Autodesk Inventor part; units mm, degrees
ref_plane "Work Plane1" through (0, -22.925, 3.175) normal (1, 0, 0) x (0, 0, -1)
ref_plane "Work Plane2" through (-20.675, -22.925, -45) normal (0, 0, -1) x (1, 0, 0)
ref_plane "YZ Plane" through (0, 0, 0) normal (1, 0, 0) x (0, 1, 0)
sketch "Sketch1" plane through (0, 0, 0) normal (0, 0, 1) x (1, 0, 0)
  circle A0 centre (0, 0) radius 14.925 construction
  line L0 (-5.7359, -22.925) -> (4.2584, -22.925) construction
  line L1 (0, -14.925) -> (3.9694, -14.925) construction
  line L2 (-17.5, 17.075) -> (17.5, 17.075)
  line L3 (17.5, 17.075) -> (17.5, -22.925)
  line L4 (17.5, -22.925) -> (-17.5, -22.925)
  line L5 (-17.5, -22.925) -> (-17.5, 17.075)
  line L6 (0, 31.425) -> (0, -35.6875)
  line L7 (20.675, 21.8375) -> (20.675, -26.1)
  line L8 (20.675, -26.1) -> (-20.675, -26.1)
  line L9 (-20.675, -26.1) -> (-20.675, 21.8375)
  line L10 (-17.5, 17.075) -> (-19.0875, 17.075)
  line L11 (-19.0875, 17.075) -> (-19.0875, 20.25)
  line L12 (17.5, 17.075) -> (19.0875, 17.075)
  line L13 (19.0875, 17.075) -> (19.0875, 20.25)
  line L14 (17.5, 20.25) -> (17.5, 21.8375)
  line L15 (-17.5, 20.25) -> (-17.5, 21.8375)
  line L16 (-19.0875, 20.25) -> (-17.5, 20.25)
  line L17 (-17.5, 21.8375) -> (-20.675, 21.8375)
  line L18 (19.0875, 20.25) -> (17.5, 20.25)
  line L19 (17.5, 21.8375) -> (20.675, 21.8375)
  line L20 (-17.5, 21.8375) -> (17.5, 21.8375)
  dimension "d0" = 29.85
  dimension "d1" = 8
  dimension "d2" = 40
  dimension "d3" = 35
  dimension "d5" = 3.175
  dimension "d6" = 3.175
  dimension "d7" = 3.175
  dimension "d10" = 3.175
  dimension "d11" = 1.5875
  dimension "d12" = 1.5875
extrude "Extrusion1" add sketch "Sketch1" against normal blind 90 contours L5 L4 L6 L8 L9 L17 L15 L16 L11 L10 | L12 L13 L18 L14 L19 L7 L8 L6 L4 L3
extrude "Extrusion2" add sketch "Sketch1" along normal blind 3.175 contours L2 L6 L4 L5 | L5 L4 L6 L8 L9 L17 L15 L16 L11 L10 | L2 L3 L4 L6 | L12 L13 L18 L14 L19 L7 L8 L6 L4 L3
sketch "Sketch2" plane through (0, 0, -90) normal (0, 0, -1) x (-1, 0, 0)
  line L0 (19.0875, 17.075) -> (17.5, 17.075)
  line L1 (17.5, 17.075) -> (17.5, -22.925)
  line L2 (17.5, -22.925) -> (-17.5, -22.925)
  line L3 (-17.5, -22.925) -> (-17.5, 17.075)
  line L4 (-17.5, 17.075) -> (-19.0875, 17.075)
  line L5 (-19.0875, 17.075) -> (-19.0875, 20.25)
  line L6 (-19.0875, 20.25) -> (-17.5, 20.25)
  line L7 (-17.5, 20.25) -> (-17.5, 21.8375)
  line L8 (-17.5, 21.8375) -> (-20.675, 21.8375)
  line L9 (-20.675, 21.8375) -> (-20.675, -26.1)
  line L10 (-20.675, -26.1) -> (20.675, -26.1)
  line L11 (20.675, -26.1) -> (20.675, 21.8375)
  line L12 (20.675, 21.8375) -> (17.5, 21.8375)
  line L13 (17.5, 21.8375) -> (17.5, 20.25)
  line L14 (17.5, 20.25) -> (19.0875, 20.25)
  line L15 (19.0875, 20.25) -> (19.0875, 17.075)
  line L16 (-17.5, 21.8375) -> (17.5, 21.8375)
  line L17 (-17.5, 20.25) -> (17.5, 20.25)
  line L18 (-17.5, 17.075) -> (17.5, 17.075)
  point P0 (0, 0)
extrude "Extrusion3" add sketch "Sketch2" along normal blind 3.175
extrude "Extrusion4" cut sketch "Sketch2" along normal blind 1.5875 contours L0 L18 L4 L5 L6 L17 L14 L15
sketch "Sketch3" plane through (-17.5, -22.925, 0) normal (0, 1, 0) x (1, 0, 0)
  line L0 (-3.175, 93.175) -> (-3.175, -3.175)
  line L1 (38.175, 93.175) -> (-3.175, 93.175)
  line L2 (38.175, 93.175) -> (38.175, -3.175)
  line L3 (-3.175, -3.175) -> (38.175, -3.175)
  line L4 (-3.175, 93.175) -> (-3.175, -3.175) construction
  line L5 (-3.175, 45) -> (38.175, 45) construction
  line L6 (38.175, 93.175) -> (38.175, -3.175) construction
  line L7 (-3.175, -3.175) -> (38.175, -3.175) construction
  line L8 (17.5, -3.175) -> (17.5, 93.175) construction
  line L9 (38.175, 93.175) -> (-3.175, 93.175) construction
  circle A0 centre (17.5, 46.03) radius 9.75
  circle A1 centre (17.5, 46.03) radius 12.75 construction
  line L10 (17.5, 58.78) -> (17.5, 55.78) construction
  line L11 (17.5, 57.28) -> (18.611, 57.28) construction
  point P0 (17.5, 0)
  dimension "d22" = 19.5
  dimension "d23" = 25.5
  dimension "d21" = 1.03
extrude "Extrusion5" cut sketch "Sketch3" against normal up to next contours A0
hole "Hole1" at (0, -22.925, -57.28) direction (0, -1, 0) diameter 2 depth 8 tip angle 118
ref_plane "Work Plane1" through (0, -22.925, 3.175) normal (1, 0, 0) x (0, 0, -1)
ref_plane "Work Plane2" through (-20.675, -22.925, -45) normal (0, 0, -1) x (1, 0, 0)
pattern_circular "Circular Pattern1" count 8 over 360 about axis through (0, -26.1, -46.03) along (0, 1, 0) of "Hole1"
sketch "Sketch4" plane through (-17.5, 21.8375, -90) normal (0, 1, 0) x (1, 0, 0)
  circle A0 centre (25.455, -36.015) radius 1
  circle A1 centre (28.75, -43.97) radius 1
  circle A2 centre (25.455, -51.925) radius 1
  circle A3 centre (17.5, -55.22) radius 1
  circle A4 centre (9.545, -51.925) radius 1
  circle A5 centre (6.25, -43.97) radius 1
  circle A6 centre (9.545, -36.015) radius 1
  circle A7 centre (17.5, -32.72) radius 1
  circle A8 centre (17.5, -43.97) radius 9.75
  line L0 (35, -90) -> (0, -90)
  line L1 (35, -90) -> (35, 0)
  line L2 (0, 0) -> (35, 0)
  line L3 (0, -90) -> (0, 0)
  line L4 (0, 0) -> (0, -93.175)
  line L5 (0, 0) -> (35, 0)
  line L6 (35, 0) -> (35, -93.175)
  line L7 (38.175, -93.175) -> (35, -93.175)
  line L8 (38.175, 3.175) -> (38.175, -93.175)
  line L9 (-3.175, 3.175) -> (38.175, 3.175)
  line L10 (-3.175, 3.175) -> (-3.175, -93.175)
  line L11 (0, -93.175) -> (-3.175, -93.175)
  circle A9 centre (-7.175, -43.97) radius 2
  line L12 (17.5, -43.97) -> (-7.175, -43.97) construction
  arc A10 (-7.175, -39.97) -> (-7.175, -47.97) centre (-7.175, -43.97) ccw
  line L13 (-7.175, -47.97) -> (-3.175, -47.97)
  line L14 (-7.175, -39.97) -> (-3.175, -39.97)
  line L15 (-3.175, 3.175) -> (-3.175, -93.175)
  point P0 (17.5, -90)
  dimension "d38" = 4
  dimension "d39" = 4
  dimension "d40" = 2
extrude "Extrusion6" add sketch "Sketch4" against normal blind 5 contours L13 A10 L14 L10
mirror "Mirror1" about plane through (0, 0, 0) normal (1, 0, 0) of "Extrusion6"
equation "\"d5\" = d4"
equation "\"d6\" = d4"
equation "\"d7\" = d4"
equation "\"d12\" = d11"
properties part number "Lead Box" material "Lead"
Source: CAD feature listing. Evaluate the final solid. Frame: model axes, mm. A direction names the side the tool comes from. Coordinates: 2 decimals unless noted, no trailing zeros. Write each loop counter-clockwise with the first axis right and the second up, starting at its lowest first coordinate (ties: lowest second). Pieces come first, ordered by that corner, then holes. Notation, with made-up numbers: (52.5, 85) -> (97.5, 85) arc R3 ccw to (97.5, 89) -> close; hole circle Ø7 at (85.25, 66.5). An arc over 180 degrees is marked (long way). Return JSON: item names as keys, results as strings. Group by question number.
1) Set-up query: faces 1 (the face through (-19.088, 19, -44)), 2 (the face through (23, 19, -42.03)), 3 (the face through (-23, 19, -42.03)), 4 (the face through (-23, 19, -50.03)). Return all of +Z, -Z, +X, -X, +Y, -Y with unobstructed straight access to the full face (end or side cutting, diameter ignored); none if empty.
2) Mould query, pull axis Y, two halves, no side actions, for faces 5 (the face through (19.088, 19, -44)), 6 (the face through (0.3, -26.1, -33.6)), 7 (the face through (-19, 21.838, -55)), 8 (the face through (-11, -25, -47)). Classes: +Y half, -Y half, draft (parallel to the pull), parting line (faces both ways), or undercut.
3) Ray query, line 1 along X through (y, z) = (-3, -16) (3 decimals); line 2 along Z through (x, y) = (4.5, 0) (3 decimals); line 3 along Y through (x, z) = (-8, -83.5) (3 decimals). Return the intervals inside material, ascending.
4) Section query C-C, the plane x = 0. State how many separate pieces and enclosed holes the cut face has, plus the area to 3 significant figures.
5) Contact query for flat-ended pins moving along their axis: P1, Ø2, axis at x = 5.5, z = -13, coming from the +Y side (3 decimals); P2, Ø0.5, axis at y = 21, z = -27.5, coming from the -X side (3 decimals); P3, Ø4, axis at x = -25.5, z = -47, coming from the -Y side; P4, Ø1.2, axis at x = 7.95, z = -38.08, coming from the -Y side. Output: stop coordinate, or through.
6) Section query D-D, the plane y = -4. Return loops of the section in (x, z) (3 decimals), plus the area to 3 significant figures.
From the geometry:
{
 "1": {"face 1": "+Z", "face 2": "+Z, +X, +Y, -Y", "face 3": "+Z, -X, +Y, -Y", "face 4": "-Z, -X, +Y, -Y"},
 "2": {"face 5": "undercut", "face 6": "-Y half", "face 7": "+Y half", "face 8": "draft"},
 "3": {"line 1": "-20.675 to -17.5, 17.5 to 20.675", "line 2": "-93.175 to -90, 0 to 3.175", "line 3": "-26.1 to -22.925"},
 "4": {"separate pieces": "4", "enclosed holes": "0", "area": "495 mm²"},
 "5": {"P1": "y = -22.925", "P2": "x = -20.675", "P3": "y = 16.84", "P4": "through"},
 "6": {"outline": "(-20.675, -93.175) -> (20.675, -93.175) -> (20.675, 3.175) -> (-20.675, 3.175) -> close; hole (-17.5, -90) -> (17.5, -90) -> (17.5, 0) -> (-17.5, 0) -> close", "area": "834 mm²"}
}
